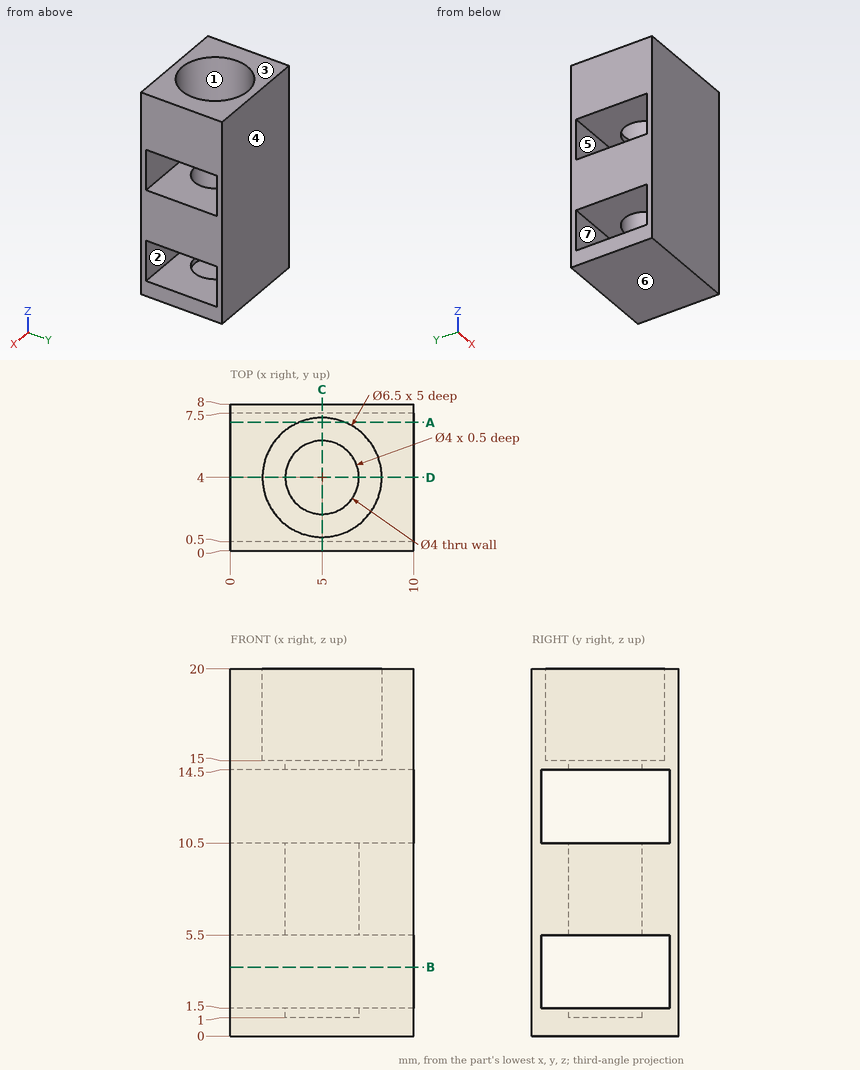
Geometry: see drawing. Coordinates: mm, zero at the bounding-box minimum. A direction names the side the tool comes from. Give positions to 0.01 mm unless a question says otherwise; leave off trailing zeros. Write each loop counter-clockwise with the first axis right and the second up, starting at its lowest first coordinate (ties: lowest second). Pieces come first, ordered by that corner, then holes. Notation, with made-up numbers: M 19.5,0 L 71.5,0 A28 ccw 71.5,22 Z; hole C -20.5,67 d8. An arc over 180 degrees is marked long. Answer in a Markdown table with one row per item. Add a question column.
(1) Section C-C on x = 5. Return loops of the section in (y, z).
(2) Mould query, pull axis Y, two halves, no side actions, for the marked faces 4, 5, 6 and 7. Classes: +Y half, -Y half, draft (parallel to the pull), parting line (faces both ways), or undercut.
(3) First-contact query: pin 1 (3 mm diameter, centred on x = 5, y = 4, fed in from +Z); pin 2 (4.5 mm diameter, centred on x = 5.5, y = 4.5, fed in from +Z). Flat tips, straight axial feed; report the tip coordinate or a pass-through.
(4) Section D-D on y = 4. Return loops of the section in (x, z).
(5) Reachability of the marked faces 1, 2 and 3 from +Z, -Z, +X, -X, +Y, -Y: full face, straight path, thin tool, end or side. Return the list, or none.
(6) Ray query, line 1 (Z direction, x = 9, y = 2.25); line 2 (Z direction, x = 6.75, y = 2.75); line 3 (Y direction, x = 5, z = 1.25). Return the intervals inside material, ascending.
(7) Section A-A on y = 7. Return loops of the section in (x, z), and give its area (4 significant figures).
(8) Section B-B on z = 3.75. Return loops of the section in (x, y), and give its area (3 significant figures).
Result set:
| question | item | result |
|---|---|---|
| 1 | outline | M 0,0 L 8,0 L 8,20 L 7.25,20 L 7.25,15 L 6,15 L 6,14.5 L 7.5,14.5 L 7.5,10.5 L 6,10.5 L 6,5.5 L 7.5,5.5 L 7.5,1.5 L 6,1.5 L 6,1 L 2,1 L 2,1.5 L 0.5,1.5 L 0.5,5.5 L 2,5.5 L 2,10.5 L 0.5,10.5 L 0.5,14.5 L 2,14.5 L 2,15 L 0.75,15 L 0.75,20 L 0,20 Z |
| 2 | face 4 | +Y half |
| 2 | face 5 | undercut |
| 2 | face 6 | draft |
| 2 | face 7 | undercut |
| 3 | pin 1 | stops at z = 1 |
| 3 | pin 2 | stops at z = 15 |
| 4 | outline | M 0,0 L 10,0 L 10,1.5 L 7,1.5 L 7,1 L 3,1 L 3,1.5 L 0,1.5 Z; M 0,5.5 L 3,5.5 L 3,10.5 L 0,10.5 Z; M 0,14.5 L 3,14.5 L 3,15 L 1.75,15 L 1.75,20 L 0,20 Z; M 7,5.5 L 10,5.5 L 10,10.5 L 7,10.5 Z; M 7,14.5 L 10,14.5 L 10,20 L 8.25,20 L 8.25,15 L 7,15 Z |
| 5 | face 1 | +Z |
| 5 | face 2 | +X, -X |
| 5 | face 3 | +Z, +X, -X, +Y, -Y |
| 6 | line 1 | z = 0 to 1.5, 5.5 to 10.5, 14.5 to 20 |
| 6 | line 2 | z = 0 to 1.5, 5.5 to 10.5, 14.5 to 15 |
| 6 | line 3 | y = 0 to 2, 6 to 8 |
| 7 | outline | M 0,0 L 10,0 L 10,1.5 L 0,1.5 Z; M 0,5.5 L 10,5.5 L 10,10.5 L 0,10.5 Z; M 0,14.5 L 10,14.5 L 10,20 L 6.25,20 L 6.25,15 L 3.75,15 L 3.75,20 L 0,20 Z |
| 7 | area | 107.5 mm^2 |
| 8 | outline | M 0,0 L 10,0 L 10,0.5 L 0,0.5 Z; M 0,7.5 L 10,7.5 L 10,8 L 0,8 Z |
| 8 | area | 10.0 mm^2 |
